from build123d import *

# Parameters (mm, degrees)
EXTRUDE1_DEPTH          = 17.5
SKETCH2_W               = 75
SKETCH2_H               = 15
CUT_EXTRUDE1_DEPTH      = 330.289006801
CUT_EXTRUDE2_DEPTH      = 327.429548295
CUT_EXTRUDE2_DEPTH_BACK = 327.429548295
SKETCH3_R               = 5


with BuildPart() as part:
    # Sketch1 → Extrude1 (new, symmetric)
    with BuildSketch(Plane.XY):
        with BuildLine():
            Line((-10, 25), (325, 25))
            Line((325, 25), (325, -25))
            Line((325, -25), (-10, -25))
            ThreePointArc((-10, -25), (-20.606601718, -20.606601718), (-25, -10))
            Line((-25, -10), (-25, 10))
            ThreePointArc((-25, 10), (-20.606601718, 20.606601718), (-10, 25))
        make_face()
    extrude(amount=EXTRUDE1_DEPTH, both=True)

    # Sketch2 → Cut-Extrude1 (cut, through all)
    with BuildSketch(Plane(origin=(0, 25, 0), x_dir=(-1, 0, 0), z_dir=(0, 1, 0))):
        with Locations((-12.5, 0)):
            Rectangle(SKETCH2_W, SKETCH2_H)
    extrude(amount=-CUT_EXTRUDE1_DEPTH, mode=Mode.SUBTRACT)

    # Sketch3 → Cut-Extrude2 (cut, two sides: drawn at the far end of the back side and taken through both)
    with BuildSketch(Plane.XY.offset(-CUT_EXTRUDE2_DEPTH_BACK)):
        Circle(SKETCH3_R)
    extrude(amount=CUT_EXTRUDE2_DEPTH + CUT_EXTRUDE2_DEPTH_BACK, mode=Mode.SUBTRACT)


solid = part.part
Can you work these out from the model? Positions are in its coordinate system, mm. A direction names the side the tool comes from. Round coordinates to 2 decimals unless told otherwise and drop trailing zeros. Write each loop counter-clockwise with the first axis right and the second up, starting at its lowest first coordinate (ties: lowest second). Pieces come first, ordered by that corner, then holes. Notation, with made-up numbers: (16.25, 35) - (36.25, 35) arc R23 ccw to (36.25, 65) - close; hole circle Ø6 at (-35.75, 24.5). An arc over 180 degrees is marked (long way). Write each question's results on one line, items separated by ' | '. Start each with the question number.
1) Please list where these lines run through material, in increasing order: line 1 (Y direction, x = 0, z = 13); line 2 (X direction, y = 0, z = 12.5); line 3 (Z direction, x = 15, y = -15.5).
2) Suppose I cut it at A-A (y = 0). List the corners of the cut face in (x, z) for me, and give its area (3 significant figures).
3) Suppose I cut it at C-C (z = 3). List the corners of the cut face in (x, y) for me, and give its area (4 significant figures).
4) Suppose I cut it at B-B (x = 0). List the corners of the cut face in (y, z) for me.
5) We'd pull the mould along Y, two halves only. Please class faces 3 (the cylindrical face through (-20.49, -20.72, 12.57)), 4 (the flat face through (325, 0, 0)), 5 (the cylindrical face through (-1.08, -4.88, -12.57)): released by +Y, released by -Y, zero draft, split by the parting line, or undercut.
6) For pin 1 Ø12 at (y, z) = (-7.5, -2) entering from -X, with a flat end and sliding along its axis, tell me the tip position at first contact or that it passes through.
7) Which directions (+Z, -Z, +X, -X, +Y, -Y) give clear straight access to the entire face, cutting with the end or side of a thin tool? Please do faces 1 (the flat face through (50, 0, 0)), 2 (the flat face through (152, 0, -17.5)).
Here are the results:
1) line 1: y = -25 to -5, 5 to 25 | line 2: x = -25 to -5, 5 to 325 | line 3: z = -17.5 to -7.5, 7.5 to 17.5
2) outline: (-25, -17.5) - (-5, -17.5) - (-5, -7.5) - (-25, -7.5) - close; (-25, 7.5) - (-5, 7.5) - (-5, 17.5) - (-25, 17.5) - close; (5, -17.5) - (325, -17.5) - (325, 17.5) - (5, 17.5) - (5, 7.5) - (50, 7.5) - (50, -7.5) - (5, -7.5) - close | area: 10,900 mm2
3) outline: (50, -25) - (325, -25) - (325, 25) - (50, 25) - close | area: 13,750 mm2
4) outline: (-25, -17.5) - (-5, -17.5) - (-5, -7.5) - (-25, -7.5) - close; (-25, 7.5) - (-5, 7.5) - (-5, 17.5) - (-25, 17.5) - close; (5, -17.5) - (25, -17.5) - (25, -7.5) - (5, -7.5) - close; (5, 7.5) - (25, 7.5) - (25, 17.5) - (5, 17.5) - close
5) face 3: released by -Y | face 4: zero draft | face 5: undercut
6) pin 1: stops at x = -25
7) face 1: -X, +Y, -Y | face 2: -Z, +X, -X, +Y, -Y
